from build123d import *

# Parameters (mm, degrees)
SKETCH_1_W      = 400
SKETCH_1_H      = 35
SKETCH_1_R      = 3.5
EXTRUDE_1_DEPTH = 5
SKETCH_2_W      = 400
SKETCH_2_H      = 5
EXTRUDE_2_DEPTH = 10
FILLET_1_SIZE   = 7
FILLET_1_SIZE_2 = 5


with BuildPart() as part:
    # 草图1 → 凸台-拉伸1 (new body)
    with BuildSketch(Plane.XY):
        with Locations((32.704402516, 130.419346185)):
            Rectangle(SKETCH_1_W, SKETCH_1_H)
        with Locations((-127.295597484, 134.919346185)):
            Circle(SKETCH_1_R, mode=Mode.SUBTRACT)
        with Locations(Location((192.704402516, 134.919346185, 0), (0, 0, 180))):
            Circle(SKETCH_1_R, mode=Mode.SUBTRACT)
    extrude(amount=EXTRUDE_1_DEPTH)

    # 草图2 → 凸台-拉伸2 (add)
    with BuildSketch(Plane(origin=(0, 0, 0), x_dir=(-1, 0, 0), z_dir=(0, 0, -1))):
        with Locations((-32.704402516, 115.419346185)):
            Rectangle(SKETCH_2_W, SKETCH_2_H)
    extrude(amount=EXTRUDE_2_DEPTH)

    # 圆角1
    # an asymmetric fillet: 7, 5 mm, written as the material it takes off along each edge
    with BuildSketch(Plane(origin=(250.204402516, 112.919346185, 5), x_dir=(0, 1, 0), z_dir=(-1, 0, 0))) as fillet_1_piece_1:
        with BuildLine():
            Bezier((FILLET_1_SIZE, 0), (0, 0), (0, FILLET_1_SIZE_2), weights=[1, 0.707106781, 1])
            Line((0, FILLET_1_SIZE_2), (0, 0))
            Line((0, 0), (FILLET_1_SIZE, 0))
        make_face()
    extrude(amount=435, mode=Mode.SUBTRACT)


solid = part.part
Source: CAD feature listing. Evaluate the final solid. Frame: model axes, mm. A direction names the side the tool comes from. Give positions to 0.01 mm unless a question says otherwise; leave off trailing zeros. Write each loop counter-clockwise with the first axis right and the second up, starting at its lowest first coordinate (ties: lowest second). Pieces come first, ordered by that corner, then holes. Notation, with made-up numbers: (32.5, 58) - (52.5, 58) arc R26 ccw to (52.5, 90) - close; hole circle Ø4 at (5, -15). An arc over 180 degrees is marked (long way). Write item = value, one per line. Start each with the question number.
Q1. Draft query along Y for faces 3 (the flat face through (36, 117.919, -5)), 4 (the flat face through (36, 112.919, -5)), 5 (the cylindrical face through (-130.073, 132.79, 2.465)), 6 (the flat face through (-167.296, 126, 1)). Return one class per face: +Y half, -Y half, draft (parallel to the pull), parting line (faces both ways), or undercut.
Q2. Material intervals for probe 1 along Y at (x, z) = (83.5, -3.25); probe 2 along Z at (x, y) = (-94, 129); probe 3 along Z at (x, y) = (-79, 115.5), sorted ascending.
Q3. Cut plane B-B, the plane z = -6.5. Return loops of the section in (x, y).
Q4. Cut plane A-A, the plane y = 144. Return loops of the section in (x, z).
Q5. Pin query (flat end, axial travel): pin 1 Ø2 at (x, z) = (33, -2.5) entering from +Y; pin 2 Ø9 at (x, y) = (30, 126.5) entering from -Z; pin 3 Ø2 at (x, y) = (11, 118.5) entering from +Z. Return the tip coordinate at first contact, or that it passes through.
Q6. Reachability of faces 1 (the flat face through (30, 133, 0)), 2 (the cylindrical face through (189.47, 136.26, 2.46)) from +Z, -Z, +X, -X, +Y, -Y: full face, straight path, thin tool, end or side. Return the list, or none.
Computed values:
q1.face_3 = +Y half
q1.face_4 = -Y half
q1.face_5 = undercut
q1.face_6 = draft
q2.probe_1 = 112.92 to 117.92
q2.probe_2 = 0 to 5
q2.probe_3 = -10 to 3.88
q3.outline = (-167.3, 112.92) - (232.7, 112.92) - (232.7, 117.92) - (-167.3, 117.92) - close
q4.outline = (-167.3, 0) - (232.7, 0) - (232.7, 5) - (-167.3, 5) - close
q5.pin_1 = 117.92
q5.pin_2 = 0
q5.pin_3 = 4.99
q6.face_1 = -Z, +X, -X, +Y
q6.face_2 = +Z, -Z
